Read the model definition and answer for the solid it produces. Units are mm, in the model's axes. Face numbers are marked on the shaded views. A direction names the side the tool comes from. Round coordinates to 2 decimals unless told otherwise and drop trailing zeros. Write each loop counter-clockwise with the first axis right and the second up, starting at its lowest first coordinate (ties: lowest second). Pieces come first, ordered by that corner, then holes. Notation, with made-up numbers: (52, 70.5) - (71, 70.5) arc R14 ccw to (71, 91.5) - close; hole circle Ø2 at (-19, 70). An arc over 180 degrees is marked (long way). Answer as CSV lines item,"result". Start each with the question number.
1) Find section D-D on x = 24. Determine the outline of the cut face in (y, z).
2) Which of the six approach directions +Z, -Z, +X, -X, +Y, -Y give full straight-line access (tool end or side, diameter ignored) to the marked faces 1, 2 and 3?
3) Find section B-B on y = 44. Determine the outline of the cut face in (x, z).
4) Find section C-C on z = 12.75. Determine the outline of the cut face in (x, y), then the cut area to 3 significant figures.
5) Find section A-A on x = 9.5. Determine the outline of the cut face in (y, z), then the cut area to 3 significant figures.
6) Consider line 1 along Y through (x, z) = (11, 10); line 2 along X through (y, z) = (22, 16); line 3 along X through (y, z) = (37, 23.75). Determine where each line is inside the solid, lowest interval first.
7) For a pull along Y with two mould halves and no side action, classify the marked faces 4, 5 and 6 as +Y half, -Y half, draft (parallel to the pull), parting line (faces both ways), or undercut.
8) This flat-tipped pin is pushed along its axis until it touches: pin 1 (4 mm diameter, centred on x = 17, z = 18.5, fed in from -Y). Where does it stop, or does it pass through?
from build123d import *

# Parameters (mm, degrees)
F1_DEPTH = 25.4


with BuildPart() as f1:
    # F0 (on Top) → F1 (new body)
    with BuildSketch(Plane.XY):
        Polygon((0, 1.544545), (0, 0), (6.723529, 0), (6.515557, 12.894255), (6.515557, 24.092648), (15.912354, 24.092648), (24.992656, 24.092648), (24.992656, 1.972236), (24.992656, 0), (32.49706, 0), (32.49706, 54.124411), (0, 54.124411), (0, 37.675023), (0, 3.922059), align=None)
        Polygon((8.740585, 33.729706), (8.740585, 46.280295), (8.740585, 47.400884), (22.860004, 47.400884), (22.860004, 33.729706), (15.912354, 33.729706), align=None, mode=Mode.SUBTRACT)
    extrude(amount=F1_DEPTH)


solid = f1.part
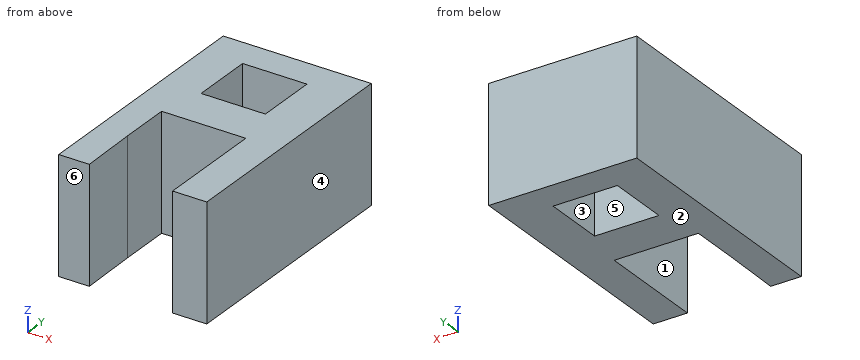
Check values:
1,outline,"(24.09, 0) - (54.12, 0) - (54.12, 25.4) - (24.09, 25.4) - close"
2,face 1,"+Z, -Z, -Y"
2,face 2,"-Z, +X, -X, +Y, -Y"
2,face 3,"+Z, -Z"
3,outline,"(0, 0) - (8.74, 0) - (8.74, 25.4) - (0, 25.4) - close; (22.86, 0) - (32.5, 0) - (32.5, 25.4) - (22.86, 25.4) - close"
4,outline,"(0, 0) - (6.72, 0) - (6.52, 12.89) - (6.52, 24.09) - (24.99, 24.09) - (24.99, 0) - (32.5, 0) - (32.5, 54.12) - (0, 54.12) - close; hole (8.74, 33.73) - (22.86, 33.73) - (22.86, 47.4) - (8.74, 47.4) - close"
4,area,"1,120 mm^2"
5,outline,"(24.09, 0) - (33.73, 0) - (33.73, 25.4) - (24.09, 25.4) - close; (47.4, 0) - (54.12, 0) - (54.12, 25.4) - (47.4, 25.4) - close"
5,area,"416 mm^2"
6,line 1,"y = 24.09 to 33.73, 47.4 to 54.12"
6,line 2,"x = 0 to 6.52, 24.99 to 32.5"
6,line 3,"x = 0 to 8.74, 22.86 to 32.5"
7,face 4,"draft"
7,face 5,"undercut"
7,face 6,"-Y half"
8,pin 1,"stops at y = 24.09"
